CAD build for the part. Positions are in the model's coordinates, mm. Coordinates: 2 decimals unless noted, no trailing zeros. Write each loop counter-clockwise with the first axis right and the second up, starting at its lowest first coordinate (ties: lowest second). Pieces come first, ordered by that corner, then holes. Notation, with made-up numbers: M -35,-25.75 L -14,-25.75 A23 cw -14,-11.75 Z; hole C 55,37 d7. An arc over 180 degrees is marked long. Put each result on its own line as item: value. Start each with the question number.
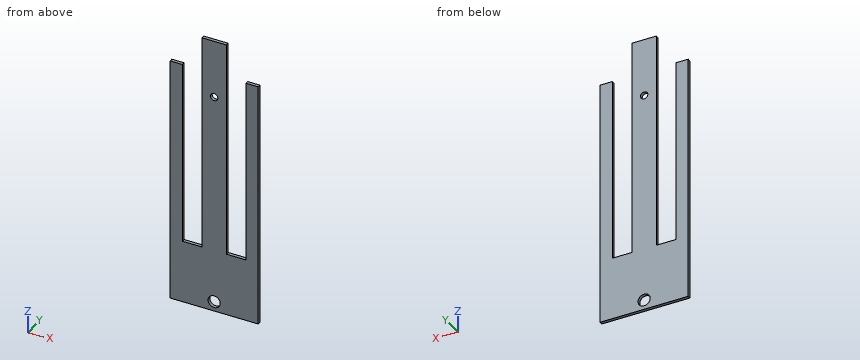
```python
from build123d import *

# Parameters (mm, degrees)
SKETCH_1_W          = 5
SKETCH_1_H          = 58
EXTRUDE_1_DEPTH     = 0.65
SKETCH_2_R          = 1.25
CUT_EXTRUDE_1_DEPTH = 10
SKETCH_3_R          = 0.75
CUT_EXTRUDE_2_DEPTH = 10


with BuildPart() as part:
    # 草图1 → 凸台-拉伸1 (new body)
    with BuildSketch(Plane(origin=(0, 0, 0), x_dir=(1, 0, 0), z_dir=(0, 1, 0))):
        Polygon((-2.5, 16), (-2.5, 29), (-9, 29), (-9, -22), (-6.5, -22), (-6.5, 16), align=None)
        Rectangle(SKETCH_1_W, SKETCH_1_H)
        Polygon((9, 29), (2.5, 29), (2.5, 16), (6.5, 16), (6.5, -22), (9, -22), align=None)
    extrude(amount=EXTRUDE_1_DEPTH)

    # 草图2 → 切除-拉伸1 (cut)
    with BuildSketch(Plane(origin=(0, 0.65, 0), x_dir=(1, 0, 0), z_dir=(0, 1, 0))):
        with Locations(Location((0, 27, 0), (0, 0, 270))):
            Circle(SKETCH_2_R)
    extrude(amount=-CUT_EXTRUDE_1_DEPTH, mode=Mode.SUBTRACT)

    # 草图3 → 切除-拉伸2 (cut)
    with BuildSketch(Plane.XZ):
        with Locations(Location((0, 17, 0), (0, 0, 270))):
            Circle(SKETCH_3_R)
    extrude(amount=-CUT_EXTRUDE_2_DEPTH, mode=Mode.SUBTRACT)


solid = part.part
```
(1) Slice it at D-D, the plane z = 17. Write the cut outline in (x, y), then the cut area to 4 significant figures.
(2) Drill centre lines: line 1 (X direction, y = 0.45, z = 17); line 2 (X direction, y = 0.5, z = -12); line 3 (X direction, y = 0.35, z = -27). Where is each one in solid material? Low to high. Write a range as [from, to].
(3) Slice it at C-C, the plane x = 0. Write the cut outline in (y, z), then the cut area to 3 significant figures.
(4) Slice it at B-B, the plane z = -27. Write the cut outline in (x, y), then the cut area to 3 significant figures.
(5) Slice it at A-A, the plane y = 0.5. Write the cut outline in (x, z).
Result set:
1. outline: M -9,0 L -6.5,0 L -6.5,0.65 L -9,0.65 Z; M -2.5,0 L -0.75,0 L -0.75,0.65 L -2.5,0.65 Z; M 0.75,0 L 2.5,0 L 2.5,0.65 L 0.75,0.65 Z; M 6.5,0 L 9,0 L 9,0.65 L 6.5,0.65 Z
1. area: 5.525 mm^2
2. line 1: x = [-9, -6.5], [-2.5, -0.75], [0.75, 2.5], [6.5, 9]
2. line 2: x = [-9, -6.5], [-2.5, 2.5], [6.5, 9]
2. line 3: x = [-9, -1.25], [1.25, 9]
3. outline: M 0,-29 L 0.65,-29 L 0.65,-28.25 L 0,-28.25 Z; M 0,-25.75 L 0.65,-25.75 L 0.65,16.25 L 0,16.25 Z; M 0,17.75 L 0.65,17.75 L 0.65,29 L 0,29 Z
3. area: 35.1 mm^2
4. outline: M -9,0 L -1.25,0 L -1.25,0.65 L -9,0.65 Z; M 1.25,0 L 9,0 L 9,0.65 L 1.25,0.65 Z
4. area: 10.1 mm^2
5. outline: M -9,-29 L 9,-29 L 9,22 L 6.5,22 L 6.5,-16 L 2.5,-16 L 2.5,29 L -2.5,29 L -2.5,-16 L -6.5,-16 L -6.5,22 L -9,22 Z; hole C 0,-27 d2.5; hole C 0,17 d1.5
